from build123d import *

# Parameters (mm, degrees)
ESQUISSE1_W                  = 26
ESQUISSE1_H                  = 62
ESQUISSE1_R                  = 2.715
BOSS_EXTRU_1_DEPTH           = 5
ENL_V_MAT_EXTRU_1_DEPTH      = 68.416615163
ENL_V_MAT_EXTRU_1_DEPTH_BACK = 60.5
CONG_3_R                     = 0.3


with BuildPart() as part:
    # Esquisse1 → Boss.-Extru.1 (new body)
    with BuildSketch(Plane.XY):
        with Locations((13, 31)):
            Rectangle(ESQUISSE1_W, ESQUISSE1_H)
        with Locations((13, 54.5)):
            Circle(ESQUISSE1_R, mode=Mode.SUBTRACT)
    extrude(amount=BOSS_EXTRU_1_DEPTH)

    # Esquisse3 → Enlèv. mat.-Extru.1 (cut, two sides: drawn at the far end of the back side and taken through both)
    with BuildSketch(Plane.XZ.offset(-ENL_V_MAT_EXTRU_1_DEPTH_BACK)):
        Polygon((3.154700538, 0), (2, 2), (2, 2.6), (8.109401077, 2.6), (8.109401077, 2), (6.954700538, 0), align=None)
        Polygon((19.045299462, 0), (17.890598923, 2), (17.890598923, 2.6), (24, 2.6), (24, 2), (22.845299462, 0), align=None)
    extrude(amount=ENL_V_MAT_EXTRU_1_DEPTH + ENL_V_MAT_EXTRU_1_DEPTH_BACK, mode=Mode.SUBTRACT)

    # Congé3
    cong_3_edges = [part.edges().sort_by_distance(p)[0] for p in [
        (3.154700538, 30.25, 0),
        (6.954700538, 30.25, 0),
        (19.045299462, 30.25, 0),
        (22.845299462, 30.25, 0),
    ]]
    fillet(cong_3_edges, radius=CONG_3_R)


solid = part.part
Can you work these out from the model? Positions are in its coordinate system, mm. A direction names the side the tool comes from. Coordinates: 2 decimals unless noted, no trailing zeros. Loops run counter-clockwise (first coordinate to the right, second up) from the corner with the lowest first, then second, coordinate; pieces in that order, holes last. Notation, with made-up numbers: (25, -19.75) - (60, -19.75) arc R18 ccw to (60, -1.75) - close; hole circle Ø6 at (53, 17.25). An arc over 180 degrees is marked (long way). Answer as a JSON object with one key per item and string values. Group by question number.
Item 1: If we mould it in two halves opening along Y, with no side actions, what happens to faces 3 (the face through (13, 0, 3)), 4 (the face through (0, 31, 2)), 5 (the face through (12.647, 57.192, 2.465))? For each: released by +Y, released by -Y, zero draft, split by the parting line, or undercut.
Item 2: If I drill on L1, parallel to X at y = 24, z = 2.2; L2, parallel to Y at x = 13, z = 4 (3 decimals); L3, parallel to X at y = 57.5, z = 0.7, over which ranges is the centre line in solid material (lowest first)? Write a range as from..to.
Item 3: If we section it at A-A (x = 13): List the corners of the cut face in (y, z) for me (3 decimals).
Item 4: If we section it at C-C (y = 29): List the corners of the cut face in (x, z) for me, plus the area to 3 significant figures.
Item 5: For pin 1 (1.8 mm diameter, centred on x = 22, y = 22.5, fed in from -Z); pin 2 (1.3 mm diameter, centred on x = 4, z = 1.5, fed in from -Y); pin 3 (3 mm diameter, centred on x = 21.5, z = 1.5, fed in from -Y), each with a flat end and sliding along its axis, tell me the tip position at first contact or that it passes through.
Item 6: On a 3-axis mill with a long thin cutter (end or side, diameter ignored), from which of +Z, -Z, +X, -X, +Y, -Y can I reach the whole of each face in a straight line? I mean faces 1 (the face through (2.454, 30.674, 1.214)), 2 (the face through (13, 31, 5)). Say none if no direction works.
Item 7: If we section it at D-D (x = 6): List the corners of the cut face in (y, z) for me, plus the area to 3 significant figures.
Returned:
{
 "1": {"face 3": "released by -Y", "face 4": "zero draft", "face 5": "undercut"},
 "2": {"L1": "x = 0..2, 8.11..17.89, 24..26", "L2": "y = 0..51.785, 57.215..62", "L3": "x = 0..2.75, 7.36..18.64, 23.25..26"},
 "3": {"outline": "(0, 0) - (51.785, 0) - (51.785, 5) - (0, 5) - close; (57.215, 0) - (62, 0) - (62, 5) - (57.215, 5) - close"},
 "4": {"outline": "(0, 0) - (2.64, 0) arc R0.3 ccw to (2.89, 0.45) - (2, 2) - (2, 2.6) - (8.11, 2.6) - (8.11, 2) - (7.21, 0.45) arc R0.3 ccw to (7.47, 0) - (18.53, 0) arc R0.3 ccw to (18.79, 0.45) - (17.89, 2) - (17.89, 2.6) - (24, 2.6) - (24, 2) - (23.11, 0.45) arc R0.3 ccw to (23.36, 0) - (26, 0) - (26, 5) - (0, 5) - close", "area": "103 mm²"},
 "5": {"pin 1": "stops at z = 2.6", "pin 2": "stops at y = 60.5", "pin 3": "stops at y = 0"},
 "6": {"face 1": "-Y", "face 2": "+Z, +X, -X, +Y, -Y"},
 "7": {"outline": "(0, 2.6) - (60.5, 2.6) - (60.5, 0) - (62, 0) - (62, 5) - (0, 5) - close", "area": "153 mm²"}
}
